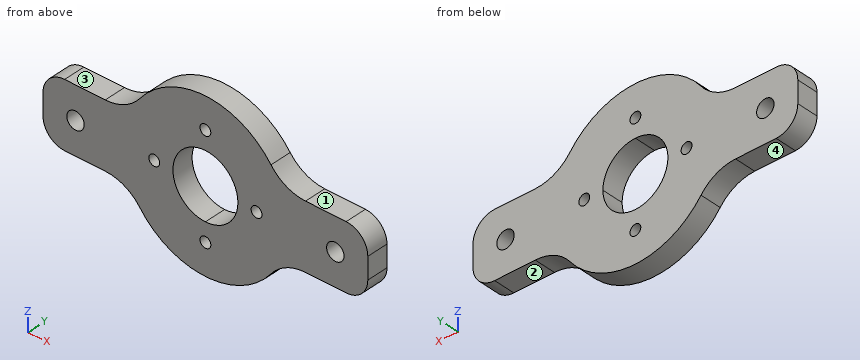
from build123d import *

# Parameters (mm, degrees)
SKETCH1_R           = 1.5875
SKETCH1_R_2         = 2.5527
BOSS_EXTRUDE2_DEPTH = 6.35


with BuildPart() as part:
    # Sketch1 → Boss-Extrude2 (new body)
    # profile 1 of 10: a face of its own
    with BuildSketch(Plane(origin=(0, 0, 0), x_dir=(1, 0, 0), z_dir=(0, 1, 0))):
        with BuildLine():
            Line((-4.5e-08, 9.525), (-22.170504618, 9.525))
            ThreePointArc((-22.170504618, 9.525), (-24.13, 0), (-22.170504618, -9.525))
            Line((-22.170504618, -9.525), (4.2e-08, -9.525))
            ThreePointArc((4.2e-08, -9.525), (-9.525, -4.4e-08), (-4.5e-08, 9.525))
        make_face()
        with Locations(Location((-15, 0, 0), (0, 0, 270))):
            Circle(SKETCH1_R, mode=Mode.SUBTRACT)
    # profile 2 of 10: a face of its own
    with BuildSketch(Plane(origin=(0, 0, 0), x_dir=(1, 0, 0), z_dir=(0, 1, 0))):
        with BuildLine():
            Line((22.170504618, 9.525), (-4.5e-08, 9.525))
            ThreePointArc((-4.5e-08, 9.525), (6.735192075, 6.735192107), (9.525, 0))
            ThreePointArc((9.525, 0), (6.735192106, -6.735192076), (4.2e-08, -9.525))
            Line((4.2e-08, -9.525), (22.170504618, -9.525))
            ThreePointArc((22.170504618, -9.525), (23.635049994, -4.86223321), (24.13, 0))
            ThreePointArc((24.13, 0), (23.635049994, 4.86223321), (22.170504618, 9.525))
        make_face()
        with Locations(Location((15, 0, 0), (0, 0, 270))):
            Circle(SKETCH1_R, mode=Mode.SUBTRACT)
    # profile 3 of 10: a face of its own
    with BuildSketch(Plane(origin=(0, 0, 0), x_dir=(1, 0, 0), z_dir=(0, 1, 0))):
        with BuildLine():
            Line((4.2e-08, -9.525), (-22.170504618, -9.525))
            ThreePointArc((-22.170504618, -9.525), (-20.858463978, -12.131833353), (-19.241313721, -14.561206897))
            ThreePointArc((-19.241313721, -14.561206897), (0, -24.13), (19.241313721, -14.561206897))
            ThreePointArc((19.241313721, -14.561206897), (20.858463978, -12.131833353), (22.170504618, -9.525))
            Line((22.170504618, -9.525), (4.2e-08, -9.525))
        make_face()
        with Locations(Location((0, -15, 0), (0, 0, 270))):
            Circle(SKETCH1_R, mode=Mode.SUBTRACT)
    # profile 4 of 10: a face of its own
    with BuildSketch(Plane(origin=(0, 0, 0), x_dir=(1, 0, 0), z_dir=(0, 1, 0))):
        with BuildLine():
            ThreePointArc((-19.241313721, 14.561206897), (-20.858463978, 12.131833353), (-22.170504618, 9.525))
            Line((-22.170504618, 9.525), (-4.5e-08, 9.525))
            Line((-4.5e-08, 9.525), (22.170504618, 9.525))
            ThreePointArc((22.170504618, 9.525), (20.858463978, 12.131833353), (19.241313721, 14.561206897))
            ThreePointArc((19.241313721, 14.561206897), (0, 24.13), (-19.241313721, 14.561206897))
        make_face()
        with Locations(Location((0, 15, 0), (0, 0, 270))):
            Circle(SKETCH1_R, mode=Mode.SUBTRACT)
    # profile 5 of 10: a face of its own
    with BuildSketch(Plane(origin=(0, 0, 0), x_dir=(1, 0, 0), z_dir=(0, 1, 0))):
        with BuildLine():
            Line((-29.368320943, 9.525), (-41.275, 9.525))
            ThreePointArc((-41.275, 9.525), (-45.765128061, 7.665128061), (-47.625, 3.175))
            Line((-47.625, 3.175), (-47.625, -3.175))
            ThreePointArc((-47.625, -3.175), (-45.765128061, -7.665128061), (-41.275, -9.525))
            Line((-41.275, -9.525), (-29.368320943, -9.525))
            Line((-29.368320943, -9.525), (-22.170504618, -9.525))
            ThreePointArc((-22.170504618, -9.525), (-24.13, 0), (-22.170504618, 9.525))
            Line((-22.170504618, 9.525), (-29.368320943, 9.525))
        make_face()
        with Locations(Location((-38.1, 0, 0), (0, 0, 270))):
            Circle(SKETCH1_R_2, mode=Mode.SUBTRACT)
    # profile 6 of 10: a face of its own
    with BuildSketch(Plane(origin=(0, 0, 0), x_dir=(1, 0, 0), z_dir=(0, 1, 0))):
        with BuildLine():
            Line((29.368320943, 9.525), (22.170504618, 9.525))
            ThreePointArc((22.170504618, 9.525), (23.635049994, 4.86223321), (24.13, 0))
            ThreePointArc((24.13, 0), (23.635049994, -4.86223321), (22.170504618, -9.525))
            Line((22.170504618, -9.525), (29.368320943, -9.525))
            Line((29.368320943, -9.525), (41.275, -9.525))
            ThreePointArc((41.275, -9.525), (45.765128061, -7.665128061), (47.625, -3.175))
            Line((47.625, -3.175), (47.625, 3.175))
            ThreePointArc((47.625, 3.175), (45.765128061, 7.665128061), (41.275, 9.525))
            Line((41.275, 9.525), (29.368320943, 9.525))
        make_face()
        with Locations(Location((38.1, 0, 0), (0, 0, 270))):
            Circle(SKETCH1_R_2, mode=Mode.SUBTRACT)
    # profile 7 of 10: a face of its own
    with BuildSketch(Plane(origin=(0, 0, 0), x_dir=(1, 0, 0), z_dir=(0, 1, 0))):
        with BuildLine():
            ThreePointArc((-19.241313721, 14.561206897), (-23.713242359, 10.853540718), (-29.368320943, 9.525))
            Line((-29.368320943, 9.525), (-22.170504618, 9.525))
            ThreePointArc((-22.170504618, 9.525), (-20.858463978, 12.131833353), (-19.241313721, 14.561206897))
        make_face()
    # profile 8 of 10: a face of its own
    with BuildSketch(Plane(origin=(0, 0, 0), x_dir=(1, 0, 0), z_dir=(0, 1, 0))):
        with BuildLine():
            ThreePointArc((-19.241313721, -14.561206897), (-20.858463978, -12.131833353), (-22.170504618, -9.525))
            Line((-22.170504618, -9.525), (-29.368320943, -9.525))
            ThreePointArc((-29.368320943, -9.525), (-23.713242359, -10.853540718), (-19.241313721, -14.561206897))
        make_face()
    # profile 9 of 10: a face of its own
    with BuildSketch(Plane(origin=(0, 0, 0), x_dir=(1, 0, 0), z_dir=(0, 1, 0))):
        with BuildLine():
            ThreePointArc((29.368320943, 9.525), (23.713242359, 10.853540718), (19.241313721, 14.561206897))
            ThreePointArc((19.241313721, 14.561206897), (20.858463978, 12.131833353), (22.170504618, 9.525))
            Line((22.170504618, 9.525), (29.368320943, 9.525))
        make_face()
    # profile 10 of 10: a face of its own
    with BuildSketch(Plane(origin=(0, 0, 0), x_dir=(1, 0, 0), z_dir=(0, 1, 0))):
        with BuildLine():
            Line((29.368320943, -9.525), (22.170504618, -9.525))
            ThreePointArc((22.170504618, -9.525), (20.858463978, -12.131833353), (19.241313721, -14.561206897))
            ThreePointArc((19.241313721, -14.561206897), (23.713242359, -10.853540718), (29.368320943, -9.525))
        make_face()
    extrude(amount=BOSS_EXTRUDE2_DEPTH)


solid = part.part
Can you work these out from the model? Positions are in its coordinate system, mm. Face numbers are marked on the shaded views. A direction names the side the tool comes from. Coordinates: 2 decimals unless noted, no trailing zeros. Write each loop counter-clockwise with the first axis right and the second up, starting at its lowest first coordinate (ties: lowest second). Pieces come first, ordered by that corner, then holes. Notation, with made-up numbers: (-24, 53) - (10, 53) arc R22 ccw to (10, 89) - close; hole circle Ø10 at (23.25, 40). An arc over 180 degrees is marked (long way). Return JSON: item names as keys, results as strings. Group by question number.
Item 1: Which directions (+Z, -Z, +X, -X, +Y, -Y) give clear straight access to the entire face, cutting with the end or side of a thin tool? Please do the marked faces 1, 2, 3 and 4.
Item 2: If we section it at B-B (y = 3.25): Count the separate pieces of the cut face and the enclosed holes in it, then the cut area to 3 significant figures.
Item 3: If we section it at C-C (z = 6): Write out the boundary of the cut face in (x, y), then the cut area to 3 significant figures.
Item 4: Please list where these lines run through material, in increasing order: probe 1 along X at (y, z) = (5.25, 0) (1 decimal); probe 2 along X at (y, z) = (3.75, -14); probe 3 along X at (y, z) = (1.25, 7).
Item 5: I'm going to push a flat-ended pin straight in: pin 1 Ø1.9 at (x, y) = (-34, 4.5) entering from -Z (3 decimals). Where does the tip first touch, or does it pass through?
Item 6: If we section it at D-D (z = -20.5): Write out the boundary of the cut face in (x, y).
Item 7: If we section it at A-A (x = -38.1): Write out the boundary of the cut face in (y, z) (3 decimals).
Return value:
{
 "1": {"face 1": "+Z, +X, +Y, -Y", "face 2": "-Z, +X, +Y, -Y", "face 3": "+Z, -X, +Y, -Y", "face 4": "-Z, -X, +Y, -Y"},
 "2": {"separate pieces": "1", "enclosed holes": "7", "area": "2,390 mm^2"},
 "3": {"outline": "(-46.96, 0) - (-7.4, 0) - (-7.4, 6.35) - (-46.96, 6.35) - close; (7.4, 0) - (46.96, 0) - (46.96, 6.35) - (7.4, 6.35) - close", "area": "502 mm^2"},
 "4": {"probe 1": "x = -47.6 to -40.7, -35.5 to -16.6, -13.4 to -9.5, 9.5 to 13.4, 16.6 to 35.5, 40.7 to 47.6", "probe 2": "x = -19.69 to -1.23, 1.23 to 19.69", "probe 3": "x = -46.34 to -6.46, 6.46 to 46.34"},
 "5": {"pin 1": "stops at z = -9.525"},
 "6": {"outline": "(-12.73, 0) - (12.73, 0) - (12.73, 6.35) - (-12.73, 6.35) - close"},
 "7": {"outline": "(0, -9.525) - (6.35, -9.525) - (6.35, -2.553) - (0, -2.553) - close; (0, 2.553) - (6.35, 2.553) - (6.35, 9.525) - (0, 9.525) - close"}
}
